The listing builds one solid part. Answer for the finished solid, in the listing's coordinates (mm). Face numbers are marked on the shaded views. A direction names the side the tool comes from. Coordinates: 2 decimals unless noted, no trailing zeros. Write each loop counter-clockwise with the first axis right and the second up, starting at its lowest first coordinate (ties: lowest second). Pieces come first, ordered by that corner, then holes.
from build123d import *
from OCP.BRepFilletAPI import BRepFilletAPI_MakeChamfer

# Parameters (mm, degrees)
BOSS_EXTRUDE1_DEPTH                             = 10
FILLET4_R                                       = 4
SKETCH8_W                                       = 16
SKETCH8_H                                       = 7
BOSS_EXTRUDE3_DEPTH                             = 2
SKETCH9_W                                       = 16
SKETCH9_H                                       = 34
BOSS_EXTRUDE4_DEPTH                             = 6
BOSS_EXTRUDE5_DEPTH                             = 10
CUT_EXTRUDE3_DEPTH                              = 10
CHAMFER1_SIZE                                   = 6
CHAMFER1_SIZE_2                                 = 9.239189783
SKETCH13_W                                      = 7
SKETCH13_H                                      = 6
BOSS_EXTRUDE6_DEPTH                             = 88
CHAMFER2_SIZE                                   = 3.5
CSK_FOR_M4_FLAT_HEAD_MACHINE_SCREW1_D           = 4
CSK_FOR_M4_FLAT_HEAD_MACHINE_SCREW1_DEPTH       = 53.798278762
CSK_FOR_M4_FLAT_HEAD_MACHINE_SCREW1_CSINK_D     = 7.6
CSK_FOR_M4_FLAT_HEAD_MACHINE_SCREW1_CSINK_ANGLE = 90
CSK_FOR_M4_FLAT_HEAD_MACHINE_SCREW1_TIP         = 1.201721238
FILLET5_R                                       = 4
SKETCH17_W                                      = 6
SKETCH17_H                                      = 1
BOSS_EXTRUDE7_DEPTH                             = 10
CUT_EXTRUDE4_DEPTH                              = 3.15
CHAMFER3_SIZE                                   = 6.3
CHAMFER3_SIZE2                                  = 9.340134102


# Some blends are built 0.0001 mm under size
with BuildPart() as part:
    # Sketch1 → Boss-Extrude1 (new body)
    with BuildSketch(Plane(origin=(0, 0, 0), x_dir=(1, 0, 0), z_dir=(0, 1, 0))):
        Polygon((0, 17), (-60, 17), (-60, 10), (-43.720595315, 10), (-36.720595315, 10), (-28, 10), (-20, 10), (0, 10), align=None)
        Polygon((60, 17), (0, 17), (0, 10), (20, 10), (28, 10), (36.720595315, 10), (43.720595315, 10), (60, 10), align=None)
        Polygon((60, -10), (51, -10), (44, -10), (44, -17), (60, -17), align=None)
        Polygon((-44, -10), (-51, -10), (-60, -10), (-60, -17), (-44, -17), align=None)
    extrude(amount=BOSS_EXTRUDE1_DEPTH)

    # Fillet4
    fillet4_edges = [part.edges().sort_by_distance(p)[0] for p in [
        (60, 10, -13.5),
        (-60, 10, -13.5),
    ]]
    fillet(fillet4_edges, radius=FILLET4_R)

    # Sketch8 → Boss-Extrude3 (add)
    with BuildSketch(Plane.XZ):
        with Locations((-52, 13.5)):
            Rectangle(SKETCH8_W, SKETCH8_H)
        with Locations((52, 13.5)):
            Rectangle(SKETCH8_W, SKETCH8_H)
        with Locations((52, -13.5)):
            Rectangle(SKETCH8_W, SKETCH8_H)
        with Locations((-52, -13.5)):
            Rectangle(SKETCH8_W, SKETCH8_H)
    extrude(amount=BOSS_EXTRUDE3_DEPTH)

    # Sketch9 → Boss-Extrude4 (add)
    with BuildSketch(Plane.XZ.offset(2)):
        with Locations((-52, 0)):
            Rectangle(SKETCH9_W, SKETCH9_H)
        with Locations((52, 0)):
            Rectangle(SKETCH9_W, SKETCH9_H)
    extrude(amount=BOSS_EXTRUDE4_DEPTH)

    # Sketch10 → Boss-Extrude5 (add)
    with BuildSketch(Plane(origin=(0, 10, 0), x_dir=(1, 0, 0), z_dir=(0, 1, 0))):
        Polygon((-33.045425071, 17), (-18.545425071, 30), (-2.545425071, 30), (11.954574929, 17), align=None)
    extrude(amount=-BOSS_EXTRUDE5_DEPTH)

    # Sketch11 → Cut-Extrude3 (cut)
    with BuildSketch(Plane(origin=(0, 10, 0), x_dir=(1, 0, 0), z_dir=(0, 1, 0))):
        with BuildLine():
            Line((-7.545425071, 25), (-7.545425071, 11))
            ThreePointArc((-7.545425071, 11), (-10.545425071, 8), (-13.545425071, 11))
            Line((-13.545425071, 11), (-13.545425071, 25))
            ThreePointArc((-13.545425071, 25), (-10.545425071, 28), (-7.545425071, 25))
        make_face()
    extrude(amount=-CUT_EXTRUDE3_DEPTH, mode=Mode.SUBTRACT)

    # Chamfer1
    chamfer1_edges_1 = [part.edges().sort_by_distance(p)[0] for p in [
        (-60, -8, 0),
    ]]
    chamfer1_side_1 = [part.faces().sort_by_distance(p)[0] for p in [
        (-60, -7.88, 0),
    ]]
    chamfer1_edges_2 = [part.edges().sort_by_distance(p)[0] for p in [
        (60, -8, 0),
    ]]
    chamfer1_side_2 = [part.faces().sort_by_distance(p)[0] for p in [
        (60, -7.88, 0),
    ]]
    chamfer1 = BRepFilletAPI_MakeChamfer(part.part.solid().wrapped)
    for e in chamfer1_edges_1:
        chamfer1.Add(CHAMFER1_SIZE - 0.0001, CHAMFER1_SIZE_2 - 0.0001, e.wrapped, chamfer1_side_1[0].wrapped)
    for e in chamfer1_edges_2:
        chamfer1.Add(CHAMFER1_SIZE - 0.0001, CHAMFER1_SIZE_2 - 0.0001, e.wrapped, chamfer1_side_2[0].wrapped)
    add(Compound.cast(chamfer1.Shape()), mode=Mode.REPLACE)  # a hair under: the kernel refuses the full size

    # Sketch13 → Boss-Extrude6 (add)
    with BuildSketch(Plane.ZY.offset(-44)):
        with Locations((13.5, -5)):
            Rectangle(SKETCH13_W, SKETCH13_H)
    extrude(amount=BOSS_EXTRUDE6_DEPTH)

    # Chamfer2
    # the kernel refuses this chamfer: 3.5 mm, written as the material it takes off along each edge
    with BuildSketch(Plane(origin=(-44, -2, -10), x_dir=(-0.9996219169112968, 0.027495876610586372, 0), z_dir=(0, 0, 1)), Plane(origin=(44, -2, 10), x_dir=(0.9996219169112968, 0.027495876610586188, 0), z_dir=(0, 0, -1))) as chamfer2_piece_1:
        Polygon((CHAMFER2_SIZE * 0.999621916911, CHAMFER2_SIZE * 0.0274958766106), (-CHAMFER2_SIZE * 0.0274958766106, CHAMFER2_SIZE * 0.999621916911), (0, 0), align=None)
    extrude(amount=20, mode=Mode.SUBTRACT)

    # CSK for M4 Flat Head Machine Screw1
    with Locations(Plane(origin=(0, 0, -17), x_dir=(-1, 0, 0), z_dir=(0, 0, -1))):
        with Locations((-55, 5), (55, 5)):
            CounterSinkHole(CSK_FOR_M4_FLAT_HEAD_MACHINE_SCREW1_D / 2, CSK_FOR_M4_FLAT_HEAD_MACHINE_SCREW1_CSINK_D / 2, depth=CSK_FOR_M4_FLAT_HEAD_MACHINE_SCREW1_DEPTH, counter_sink_angle=CSK_FOR_M4_FLAT_HEAD_MACHINE_SCREW1_CSINK_ANGLE)
            with Locations((0, 0, -(CSK_FOR_M4_FLAT_HEAD_MACHINE_SCREW1_DEPTH + CSK_FOR_M4_FLAT_HEAD_MACHINE_SCREW1_TIP / 2))):  # 118° drill point
                Cone(0, CSK_FOR_M4_FLAT_HEAD_MACHINE_SCREW1_D / 2, CSK_FOR_M4_FLAT_HEAD_MACHINE_SCREW1_TIP, mode=Mode.SUBTRACT)

    # Fillet5
    fillet5_edges = [part.edges().sort_by_distance(p)[0] for p in [
        (-60, 10, 13.5),
        (60, 10, 13.5),
    ]]
    fillet(fillet5_edges, radius=FILLET5_R)

    # Sketch17 → Boss-Extrude7 (add)
    with BuildSketch(Plane(origin=(0, 10, 0), x_dir=(1, 0, 0), z_dir=(0, 1, 0))):
        with Locations((-10.545425071, 10.5)):
            Rectangle(SKETCH17_W, SKETCH17_H)
    extrude(amount=-BOSS_EXTRUDE7_DEPTH)

    # Sketch18 → Cut-Extrude4 (cut)
    with BuildSketch(Plane.XY.offset(17)):
        Polygon((51.016283143, 5), (53.008141571, 1.55), (56.991858429, 1.55), (58.983716857, 5), (56.991858429, 8.45), (53.008141571, 8.45), align=None)
        Polygon((-51.016283143, 5), (-53.008141571, 8.45), (-56.991858429, 8.45), (-58.983716857, 5), (-56.991858429, 1.55), (-53.008141571, 1.55), align=None)
    extrude(amount=-CUT_EXTRUDE4_DEPTH, mode=Mode.SUBTRACT)

    # Chamfer3: one chamfer whose edges measure the first distance from different faces: ONE call of the kernel's chamfer builder (chamfer() names one face for all edges)
    chamfer3_edges_1 = [part.edges().sort_by_distance(p)[0] for p in [
        (-44, 10, 13.5),
    ]]
    chamfer3_side_1 = [part.faces().sort_by_distance(p)[0] for p in [
        (-50, 10, 13.5),
    ]]
    chamfer3_edges_2 = [part.edges().sort_by_distance(p)[0] for p in [
        (44, 10, 13.5),
    ]]
    chamfer3_side_2 = [part.faces().sort_by_distance(p)[0] for p in [
        (50, 10, 13.5),
    ]]
    chamfer3 = BRepFilletAPI_MakeChamfer(part.part.solid().wrapped)
    for e in chamfer3_edges_1:
        chamfer3.Add(CHAMFER3_SIZE, CHAMFER3_SIZE2, e.wrapped, chamfer3_side_1[0].wrapped)  # the first distance lies on this face
    for e in chamfer3_edges_2:
        chamfer3.Add(CHAMFER3_SIZE, CHAMFER3_SIZE2, e.wrapped, chamfer3_side_2[0].wrapped)  # the first distance lies on this face
    add(Compound.cast(chamfer3.Shape()), mode=Mode.REPLACE)


solid = part.part
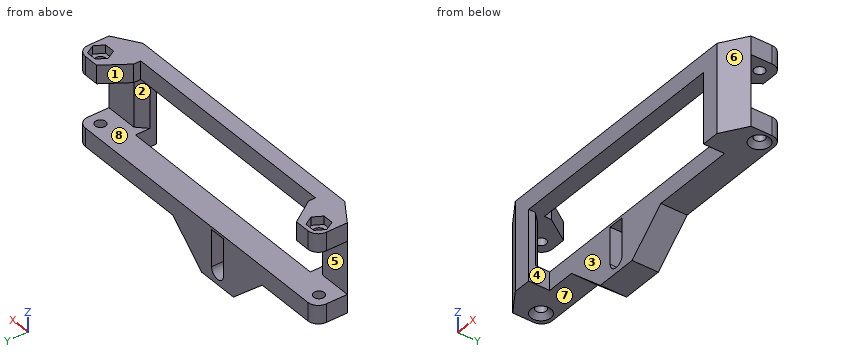
Q1. The part is cut by section A-A, the plane x = 28. Write down the section's boundary in (y, z).
Answers below:
outline: (-8, 10) - (-2, 10) - (-2, 17) - (-8, 17) - close; (0, -17) - (10, -17) - (10, -10) - (0, -10) - close
Q2. Given pin 1 (8 mm diameter, centred on y = -4, z = -19.5, fed in from -X); pin 2 (8 mm diameter, centred on x = -18, z = 7.5, fed in from +Y); pin 3 (9 mm diameter, centred on x = -44.5, y = -1, fed in from -Z); pin 4 (22 mm diameter, centred on x = 8, z = -24.5, fed in from -Y), each flat-ended and moving along its own axis, determine where each tip first touches the part or whether it passes through.
Answers below:
pin 1: stops at x = -60
pin 2: stops at y = -2
pin 3: stops at z = -17
pin 4: stops at y = 0
Q3. The part is cut by section C-C, the plane z = -21. Write down the section's boundary in (x, y).
Answers below:
outline: (-28.58, 0) - (-13.55, 0) - (-13.55, 10) - (-28.58, 10) - close; (-7.55, 0) - (7.49, 0) - (7.49, 10) - (-7.55, 10) - close
Q4. Which of the six approach directions +Z, -Z, +X, -X, +Y, -Y give full straight-line access (tool end or side, diameter ignored) to the marked faces 1, 2, 3 and 4?
Answers below:
face 1: +Z, +Y
face 2: +Y
face 3: +Z, -Z, -Y
face 4: -Z, -Y
Q5. The part is cut by section D-D, the plane y = -3.5. Write down the section's boundary in (x, z).
Answers below:
outline: (-57.69, -17) - (-44, -17) - (-44, -10) - (-46, -10) - (-46, 10) - (46, 10) - (46, -10) - (44, -10) - (44, -17) - (57.69, -17) - (57.69, 17) - (-57.69, 17) - close
Q6. Determine the mould class of the marked faces 5, 6, 7 and 8 for opening direction Z: released by +Z, released by -Z, zero draft, split by the parting line, or undercut.
Answers below:
face 5: undercut
face 6: zero draft
face 7: released by -Z
face 8: undercut
Q7. Find the intervals of material crossed by probe 1 along X at (y, z) = (5, -13.3); probe 2 along Z at (x, y) = (47, 0); probe 3 along Z at (x, y) = (13.5, 3.25), in increasing order.
Answers below:
probe 1: x = -60 to -57, -53 to -13.55, -7.55 to 53, 57 to 60
probe 2: z = -17 to -10, 10 to 17
probe 3: z = -17 to -10
